The model under review builds one solid part; all positions refer to its coordinate system, in mm. A direction names the side the tool comes from. Give positions to 0.01 mm unless a question says otherwise; leave off trailing zeros. Loops run counter-clockwise (first coordinate to the right, second up) from the corner with the lowest first, then second, coordinate; pieces in that order, holes last. Notation, with made-up numbers: M 49.25,-26.75 L 78.25,-26.75 A19 ccw 78.25,-11.75 Z; hole C 63.5,84.25 d11. An arc over 180 degrees is marked long. Return JSON: item names as keys, results as strings.
Autodesk Inventor part; units mm, degrees
ref_plane "YZ Plane" through (0, 0, 0) normal (1, 0, 0) x (0, 1, 0)
ref_plane "XZ Plane" through (0, 0, 0) normal (0, 1, 0) x (-1, 0, 0)
ref_plane "XY Plane" through (0, 0, 0) normal (0, 0, 1) x (1, 0, 0)
sketch "Sketch1" plane through (0, 0, 0) normal (0, 0, 1) x (1, 0, 0)
  circle A0 centre (0, 0) radius 2.5
  dimension "d0" = 5
extrude "Extrusion1" add sketch "Sketch1" along normal blind 200
sketch "Sketch2" plane through (0, 0, 200) normal (0, 0, 1) x (1, 0, 0)
  circle A0 centre (0, 0) radius 2.5
  circle A1 centre (0, 0) radius 1
  dimension "d3" = 2
extrude "Extrusion2" add sketch "Sketch2" along normal blind 3 contours A1
sketch "Sketch3" plane through (0, 0, 0) normal (0, 0, -1) x (-1, 0, 0)
  circle A0 centre (0, 0) radius 1
  dimension "d6" = 2
extrude "Extrusion3" add sketch "Sketch3" along normal blind 3
properties part number "Bone-20cm"
1) Consider section A-A on x = 0. Write out the cut boundary in (y, z), then the cut area to 3 significant figures.
From the geometry:
{"outline": "M -2.5,0 L -1,0 L -1,-3 L 1,-3 L 1,0 L 2.5,0 L 2.5,200 L 1,200 L 1,203 L -1,203 L -1,200 L -2.5,200 Z", "area": "1,010 mm²"}
2) Tool access review of faces 1 (the face through (-0.54, 2.44, 98.6)), 2 (the face through (1, -1, 0)), 3 (the face through (1, -1, 200)): name each direction out of +Z, -Z, +X, -X, +Y, -Y from which nothing blocks a thin tool from reaching the whole face with its end or side.
From the geometry:
{"face 1": "+Z, -Z", "face 2": "-Z", "face 3": "+Z"}
3) Insertion check: pin 1 (1 mm diameter, centred on y = -1.5, z = 92, fed in from -X). The pin has a flat end and moves straight along its axis. Give the tip position at first contact, or say it passes through.
From the geometry:
{"pin 1": "x = -2.29"}
4) Wall thickness on L1, parallel to Z at x = -0.85, y = 0.6; L2, parallel to X at y = -0.45, z = 150.5; L3, parallel to Y at x = -0.2, z = 120: over which ranges is each line inside the solid? List them lowest first. Write a range as from..to.
From the geometry:
{"L1": "0..200", "L2": "-2.46..2.46", "L3": "-2.49..2.49"}
5) Consider section C-C on z = 164. Write out the cut boundary in (x, y).
From the geometry:
{"outline": "C 0,0 d5"}
